Check sheet for the modelled part. Datum: model origin and axes. Units: mm. Face numbers are marked on the shaded views. A direction names the side the tool comes from. Coordinates: 2 decimals unless noted, no trailing zeros. Loops run counter-clockwise (first coordinate to the right, second up) from the corner with the lowest first, then second, coordinate; pieces in that order, holes last. Notation, with made-up numbers: (-20, 47.25) - (13, 47.25) arc R32 ccw to (13, 82.25) - close; hole circle Ø10 at (10, 15). An arc over 180 degrees is marked (long way). Use a Markdown table: item, result. Add a question column.
1) Sectioned sample at A-A, the plane x = 3.5. Enter the section's corners in (y, z).
2) Go/stop test with flat-tipped pins: P1, Ø2, axis at x = 1, z = 2.5, coming from the +Y side; P2, Ø4, axis at x = 7.5, z = 4, coming from the +Y side; P3, Ø1.5, axis at x = 5.5, y = 3, coming from the -Z side. Record where each tip stops, or that it passes through.
3) Draft check along Z on the marked faces 1, 2 and 3. Enter one of: pulls with the +Z half, pulls with the -Z half, needs draft (parallel to the pull), parting line crosses it, or undercut.
4) Thickness scan on line 1 (Z direction, x = 2.25, y = 0); line 2 (X direction, y = 1, z = 4.5); line 3 (Z direction, x = 1.25, y = -2). Record the ranges inside material, lowest first.
5) Tool access check on the marked faces 4, 5 and 6. Record the directions out of +Z, -Z, +X, -X, +Y, -Y that give a thin tool (end or side, any length) a straight path to the whole face; none if there is none.
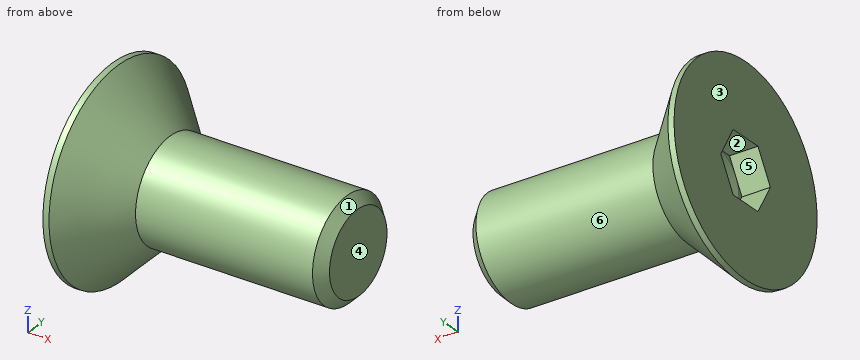
Autodesk Inventor part; units mm, degrees
ref_plane "dummy_to_bolt_XY" through (0, 0, 0) normal (1, 0, 0) x (0, 0, -1)
ref_plane "dummy_to_bolt_YZ" through (0, 0, 0) normal (0, 0, -1) x (0, 1, 0)
ref_plane "dummy_to_bolt_ZX" through (0, 0, 0) normal (0, 1, 0) x (1, 0, 0)
sketch "Sketch_1" plane through (0, 0, 0) normal (0, 0, 1) x (1, 0, 0)
  line L0 (9.2, 0) -> (0, 0)
  line L1 (-2.8, 0) -> (-2.8, 5)
  line L2 (-2.8, 5) -> (-2.5, 5)
  line L3 (-2.5, 5) -> (0, 2.5)
  line L4 (0, 2.5) -> (8.7095, 2.5)
  line L5 (8.7095, 2.5) -> (9.2, 2.0095)
  line L6 (9.2, 2.0095) -> (9.2, 0)
  line L7 (9.2, 0) -> (-2.8, 0)
revolve "Revolution1" add sketch "Sketch_1" angle 360 about axis through (9.2, 0, 0) along (1, 0, 0)
thread "Thread1"
sketch "Sketch_4" plane through (0, 0, 0) normal (0, 0, 1) x (1, 0, 0)
  line L0 (-0.9981, 0) -> (-2.8, 0)
  line L1 (-2.8, 0) -> (-2.8, 1.5)
  line L2 (-2.8, 1.5) -> (-1.4, 1.5)
  line L3 (-1.4, 1.5) -> (-0.9981, 0)
  line L4 (-0.9981, 0) -> (-2.8, 0)
revolve "Revolution2" cut sketch "Sketch_4" angle 360 about axis through (-0.9981, 0, 0) along (1, 0, 0)
sketch "Sketch_3" plane through (-2.8, 0, 0) normal (1, 0, 0) x (0, 0, -1)
  line L0 (-1.5, 0.866) -> (-1.5, -0.866)
  line L1 (-1.5, -0.866) -> (0, -1.7321)
  line L2 (0, -1.7321) -> (1.5, -0.866)
  line L3 (1.5, -0.866) -> (1.5, 0.866)
  line L4 (1.5, 0.866) -> (0, 1.7321)
  line L5 (0, 1.7321) -> (-1.5, 0.866)
extrude "Extrusion1" cut sketch "Sketch_3" along normal blind 1.4
ref_plane "dummy_to_bolt_XY" through (0, 0, 0) normal (1, 0, 0) x (0, 0, -1)
ref_plane "dummy_to_bolt_YZ" through (0, 0, 0) normal (0, 0, -1) x (0, 1, 0)
ref_plane "dummy_to_bolt_ZX" through (0, 0, 0) normal (0, 1, 0) x (1, 0, 0)
ref_plane "bolt_to_nut_XY" through (9.2, 0, 0) normal (1, 0, 0) x (0, 0, -1)
ref_plane "bolt_to_nut_YZ" through (9.2, 0, 0) normal (0, 0, -1) x (0, 1, 0)
ref_plane "bolt_to_nut_ZX" through (9.2, 0, 0) normal (0, 1, 0) x (1, 0, 0)
properties part number "SHFBS5-12"
Solved:
| question | item | result |
|---|---|---|
| 1 | outline | circle Ø5 at (0, 0) |
| 2 | P1 | stops at y = 2 |
| 2 | P2 | stops at y = 1.5 |
| 2 | P3 | stops at z = -1.09 |
| 3 | face 1 | parting line crosses it |
| 3 | face 2 | undercut |
| 3 | face 3 | needs draft |
| 4 | line 1 | z = -2.5 to 2.5 |
| 4 | line 2 | x = -2.8 to -2.11 |
| 4 | line 3 | z = -1.5 to 1.5 |
| 5 | face 4 | +Z, -Z, +X, +Y, -Y |
| 5 | face 5 | -X |
| 5 | face 6 | +X |
